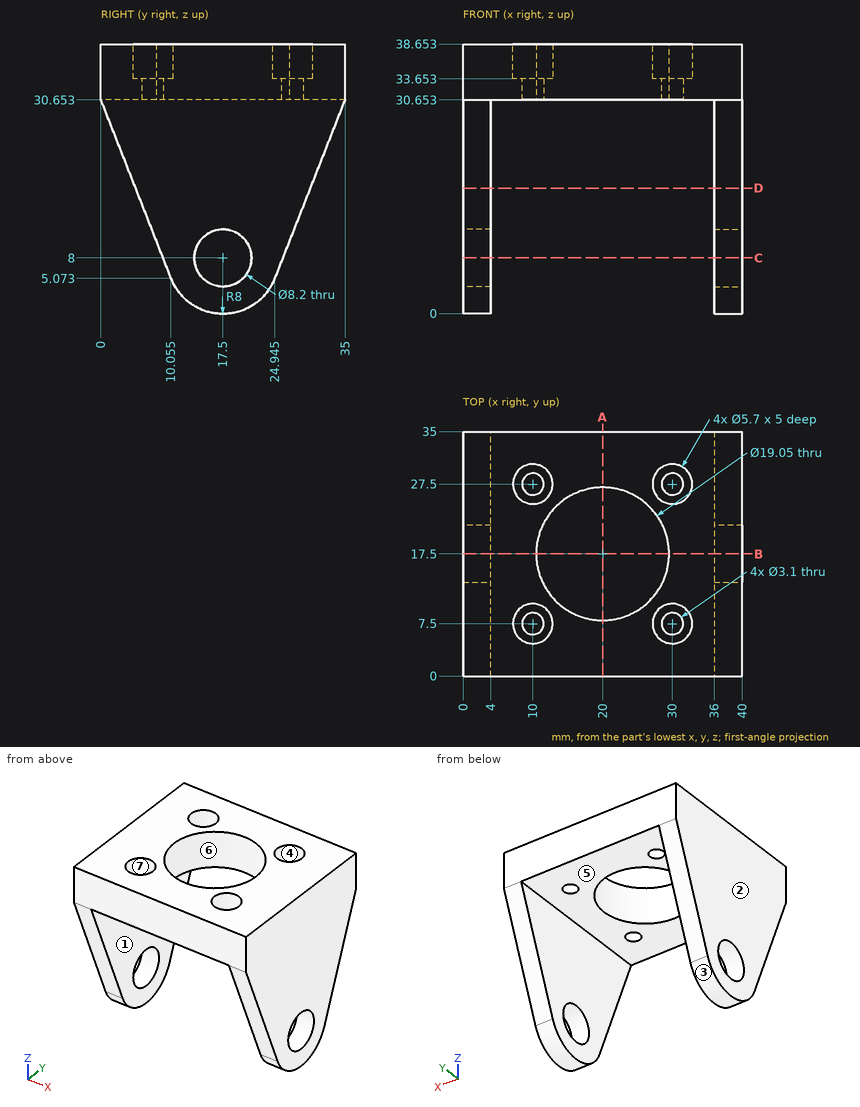
The figure shows three views and two pictorial views of one solid part (mm, origin at its lowest corner). Answer the questions. A direction names the side the tool comes from. Coordinates: 2 decimals unless noted, no trailing zeros. Loops run counter-clockwise (first coordinate to the right, second up) from the corner with the lowest first, then second, coordinate; pieces in that order, holes last.
1) Find section D-D on z = 18. Write down the section's boundary in (x, y).
2) Find section B-B on y = 17.5. Write down the section's boundary in (x, z) (1 decimal).
3) A tool of negligible diameter and unlimited length cuts with its end or side. For the marked faces 5, 6 and 7, from which of +Z, -Z, +X, -X, +Y, -Y can it reach the whole face along a straight path? Write none if from no direction.
4) Flat-ended cylindrical pins translate along their axes: pin 1 Ø4 at (x, y) = (30, 7.5) entering from +Z; pin 2 Ø4.5 at (x, y) = (10, 27.5) entering from -Z. Find the tip coordinate at first contact, or state that the pin passes through.
5) Find section C-C on z = 8. Write down the section's boundary in (x, y) (1 decimal).
6) Find the intervals of material crossed by L1, parallel to Y at x = 10, z = 37; L2, parallel to Y at x = 10, z = 32; L3, parallel to X at y = 12.5, z = 13.5, in increasing order.
7) Find section A-A on x = 20. Write down the section's boundary in (y, z) (1 decimal), then the cut area to 3 significant figures.
8) Determine the mould class of the marked faces 1, 2, 3 and 4 for opening direction X: pulls with the +X half, pulls with the -X half, needs draft (parallel to the pull), parting line crosses it, or undercut.
Values:
1. outline: (0, 4.97) - (4, 4.97) - (4, 30.03) - (0, 30.03) - close; (36, 4.97) - (40, 4.97) - (40, 30.03) - (36, 30.03) - close
2. outline: (0, 0) - (4, 0) - (4, 3.9) - (0, 3.9) - close; (0, 12.1) - (4, 12.1) - (4, 30.7) - (10.5, 30.7) - (10.5, 38.7) - (0, 38.7) - close; (29.5, 30.7) - (36, 30.7) - (36, 12.1) - (40, 12.1) - (40, 38.7) - (29.5, 38.7) - close; (36, 0) - (40, 0) - (40, 3.9) - (36, 3.9) - close
3. face 5: -Z, +Y, -Y
3. face 6: +Z, -Z
3. face 7: +Z
4. pin 1: stops at z = 33.65
4. pin 2: stops at z = 30.65
5. outline: (0, 8.9) - (4, 8.9) - (4, 13.4) - (0, 13.4) - close; (0, 21.6) - (4, 21.6) - (4, 26.1) - (0, 26.1) - close; (36, 8.9) - (40, 8.9) - (40, 13.4) - (36, 13.4) - close; (36, 21.6) - (40, 21.6) - (40, 26.1) - (36, 26.1) - close
6. L1: y = 0 to 4.65, 10.35 to 24.65, 30.35 to 35
6. L2: y = 0 to 5.95, 9.05 to 25.95, 29.05 to 35
6. L3: x = 0 to 4, 36 to 40
7. outline: (0, 30.7) - (8, 30.7) - (8, 38.7) - (0, 38.7) - close; (27, 30.7) - (35, 30.7) - (35, 38.7) - (27, 38.7) - close
7. area: 128 mm2
8. face 1: undercut
8. face 2: pulls with the -X half
8. face 3: needs draft
8. face 4: undercut
